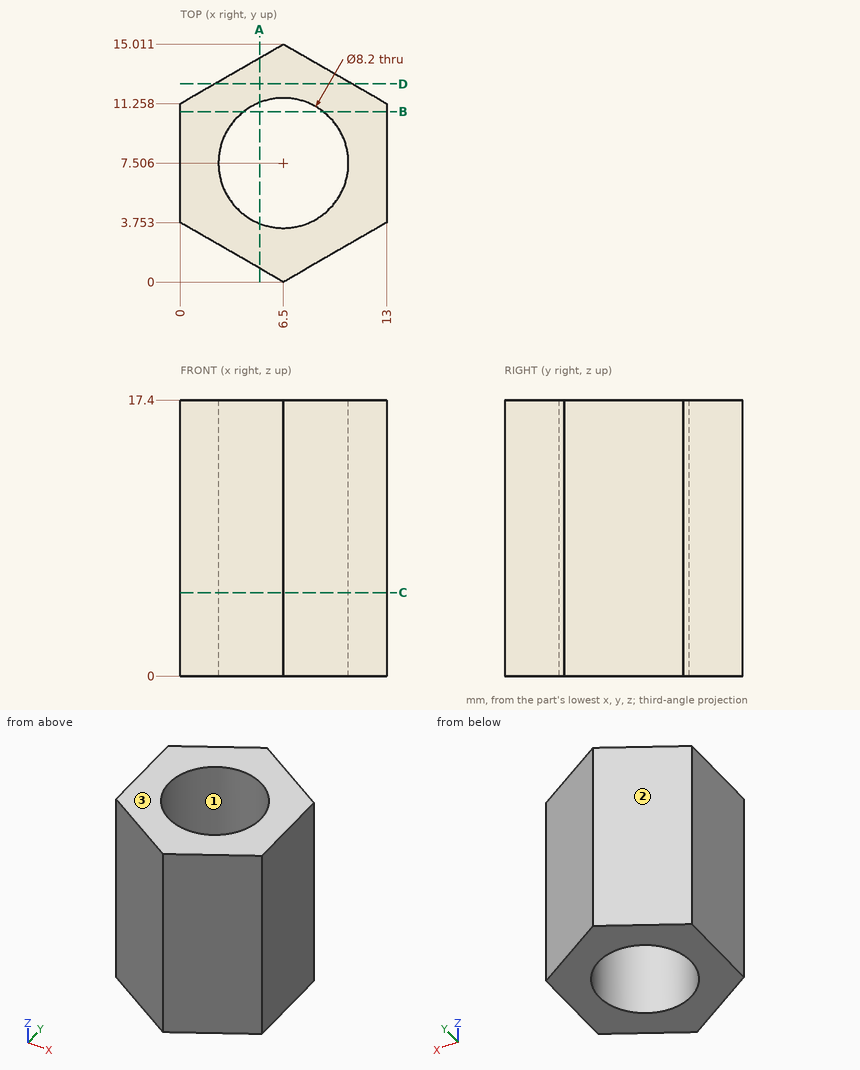
Part print with two shaded views. Sizes in mm from the minimum x, y, z corner. Give positions to 0.01 mm unless a question says otherwise; leave off trailing zeros. Write each loop counter-clockwise with the first axis right and the second up, starting at its lowest first coordinate (ties: lowest second). Pieces come first, ordered by that corner, then holes.
1) Cut at A-A on x = 5. Write the cut outline in (y, z) (1 decimal).
Resolved:
outline: (0.9, 0) - (3.7, 0) - (3.7, 17.4) - (0.9, 17.4) - close; (11.3, 0) - (14.1, 0) - (14.1, 17.4) - (11.3, 17.4) - close
2) Cut at B-B on y = 10.75. Write the cut outline in (x, z), then the cut area to 3 significant figures.
Resolved:
outline: (0, 0) - (3.99, 0) - (3.99, 17.4) - (0, 17.4) - close; (9.01, 0) - (13, 0) - (13, 17.4) - (9.01, 17.4) - close
area: 139 mm2
3) Pin check, flat tips, straight feed: pin 1 (6 mm diameter, centred on x = 6.5, z = 5, fed in from +Y); pin 2 (2 mm diameter, centred on x = 9, z = 4.5, fed in from +Y) (1 decimal); pin 3 (5 mm diameter, centred on x = 3, z = 12.5, fed in from +Y). Stop position of each tip, or through.
Resolved:
pin 1: stops at y = 15.01
pin 2: stops at y = 14.1
pin 3: stops at y = 14.43
4) Cut at D-D on y = 12.5. Write the cut outline in (x, z), then the cut area to 3 significant figures.
Resolved:
outline: (2.15, 0) - (10.85, 0) - (10.85, 17.4) - (2.15, 17.4) - close
area: 151 mm2
5) Two-plate mould, pull along X, no slides. Class the marked faces 1, 2 and 3: released by +X, released by -X, zero draft, split by the parting line, or undercut.
Resolved:
face 1: undercut
face 2: released by -X
face 3: zero draft
6) Probe L1, parallel to X at y = 5, z = 12 (1 decimal); L2, parallel to X at y = 7, z = 14.25; L3, parallel to Y at x = 3.5, z = 6.5. List the from-to ranges inside material, lowest first.
Resolved:
L1: x = 0 to 3.3, 9.7 to 13
L2: x = 0 to 2.43, 10.57 to 13
L3: y = 1.73 to 4.71, 10.3 to 13.28
7) Cut at C-C on z = 5.25. Write the cut outline in (x, y) (1 decimal).
Resolved:
outline: (0, 3.8) - (6.5, 0) - (13, 3.8) - (13, 11.3) - (6.5, 15) - (0, 11.3) - close; hole circle Ø8.2 at (6.5, 7.5)
